The model under review builds one solid part; all positions refer to its coordinate system, in mm. A direction names the side the tool comes from. Coordinates: 2 decimals unless noted, no trailing zeros. Loops run counter-clockwise (first coordinate to the right, second up) from the corner with the lowest first, then second, coordinate; pieces in that order, holes last. Notation, with made-up numbers: (-22.75, 23) - (16.25, 23) arc R15 ccw to (16.25, 31) - close; hole circle Ø5 at (55, 0.5). An arc over 180 degrees is marked (long way). Use a Markdown table: item, result. Add a question column.
1) Add section C-C, the plane y = -40.5. Give the boundary of the cut face in (x, z), and give its area (3 significant figures).
2) For faces 1 (the flat face through (112.925, -25, -24)), 2 (the flat face through (21, -15.064, -31)), 3 (the flat face through (21, -41, -64.839)), list the 3-axis set-ups (+Z, -Z, +X, -X, +Y, -Y) from which the entire face can be reached by the end or side of a thin tool; tool diameter is ignored.
3) Add section B-B, the plane z = -24.5. Give the boundary of the cut face in (x, y), and give its area (3 significant figures).
4) To check wall thickness, follow L1, parallel to Y at x = 69.5, z = -77.5; L2, parallel to Z at x = 79.5, y = -7.5; L3, parallel to Y at x = 93, z = 27.5. State the ranges of each line that lie inside material, in increasing order. Write a range as [from, to].
5) Clearance check with flat-ended pins moving along their axes: pin 1 (6 mm diameter, centred on x = -35.5, z = -49.5, fed in from +Y); pin 2 (6 mm diameter, centred on y = -37, z = -55, fed in from +X); pin 3 (12 mm diameter, centred on y = -32.5, z = 8, fed in from -X); pin 4 (6 mm diameter, centred on x = -15.5, y = -37, fed in from +Z). State where each tip first meets the part, or that it passes through.
6) Add section A-A, the plane x = 73. Give the boundary of the cut face in (y, z).
```python
from build123d import *

# Parameters (mm, degrees)
F0_W     = 185.6282874942
F0_H     = 120.2967502177
F1_DEPTH = 51.054
F2_W     = 19.7645789781
F2_H     = 101.9291467965
F3_DEPTH = 220.218
F4_W     = 15.0644443929
F4_H     = 105.4227072746
F5_DEPTH = 191.262


with BuildPart() as f1:
    # F0 (on Front) → F1 (new body)
    with BuildSketch(Plane.XZ):
        with Locations((20.1111845672, -23.0586882681)):
            Rectangle(F0_W, F0_H)
    extrude(amount=F1_DEPTH)

    # F2 (on face) → F3 (cut)
    with BuildSketch(Plane.YZ.offset(112.9253283143)):
        with Locations((-41.171710511, -13.8748865575)):
            Rectangle(F2_W, F2_H)
    extrude(amount=-F3_DEPTH, mode=Mode.SUBTRACT)

    # F4 (on face) → F5 (cut)
    with BuildSketch(Plane.YZ.offset(112.9253283143)):
        with Locations((-7.5322221965, -30.4957097396)):
            Rectangle(F4_W, F4_H)
    extrude(amount=-F5_DEPTH, mode=Mode.SUBTRACT)


solid = f1.part
```
From the geometry:
| question | item | result |
|---|---|---|
| 1 | outline | (-72.7, -83.21) - (112.93, -83.21) - (112.93, -64.84) - (-72.7, -64.84) - close |
| 1 | area | 3,410 mm^2 |
| 2 | face 1 | +Z, -Z, +X, +Y, -Y |
| 2 | face 2 | -Z, +X, -X, +Y |
| 2 | face 3 | +Z, +X, -X, -Y |
| 3 | outline | (-72.7, -31.29) - (112.93, -31.29) - (112.93, -15.06) - (-72.7, -15.06) - close |
| 3 | area | 3,010 mm^2 |
| 4 | L1 | y = [-51.05, -15.06] |
| 4 | L2 | z = [22.22, 37.09] |
| 4 | L3 | y = [-31.29, 0] |
| 5 | pin 1 | stops at y = -15.06 |
| 5 | pin 2 | passes through |
| 5 | pin 3 | stops at x = -72.7 |
| 5 | pin 4 | stops at z = -64.84 |
| 6 | outline | (-51.05, -83.21) - (-15.06, -83.21) - (-15.06, 22.22) - (0, 22.22) - (0, 37.09) - (-31.29, 37.09) - (-31.29, -64.84) - (-51.05, -64.84) - close |
